Input: dimensioned drawing with shaded views. Units: mm. Origin: part minimum x, y, z. A direction names the side the tool comes from. Round coordinates to 2 decimals unless told otherwise and drop trailing zeros. Write each loop counter-clockwise with the first axis right and the second up, starting at its lowest first coordinate (ties: lowest second). Pieces come first, ordered by that corner, then holes. Notation, with made-up numbers: M 87.25,13.5 L 145.25,13.5 A23 cw 145.25,49.5 Z; hole C 65,81 d10. An arc over 180 degrees is marked long. Answer in a Markdown table with one row per item. Add a question column.
Item 1: Cut plane D-D on x = 21. Return loops of the section in (y, z).
Item 2: Contact query for flat-ended pins moving along their axis: pin 1 (1.5 mm diameter, centred on x = 55, y = 12.5, fed in from -Z); pin 2 (7 mm diameter, centred on y = 5, z = 24, fed in from -X); pin 3 (3 mm diameter, centred on x = 2, z = 3.5, fed in from -Y); pin 4 (3 mm diameter, centred on y = 1.5, z = 28, fed in from +X). Output: stop coordinate, or through.
Item 3: Mould query, pull axis X, two halves, no side actions, for the marked faces 1, 2 and 3. Classes: released by +X, released by -X, zero draft, split by the parting line, or undercut.
Item 4: Cut plane A-A on z = 30. Return loops of the section in (x, y).
Item 5: Cut plane C-C on y = 8.5. Return loops of the section in (x, z), and give its area (3 significant figures).
Item 6: Material intervals for probe 1 along Z at (x, y) = (3, 11.85); probe 2 along X at (y, z) = (11, 35); probe 3 along Z at (x, y) = (37, 5), sorted ascending.
Item 7: Set-up query: the marked faces 4 and 5. Return all of +Z, -Z, +X, -X, +Y, -Y with unobstructed straight access to the full face (end or side cutting, diameter ignored); none if empty.
Item 8: Cut plane B-B on x = 3. Return loops of the section in (y, z).
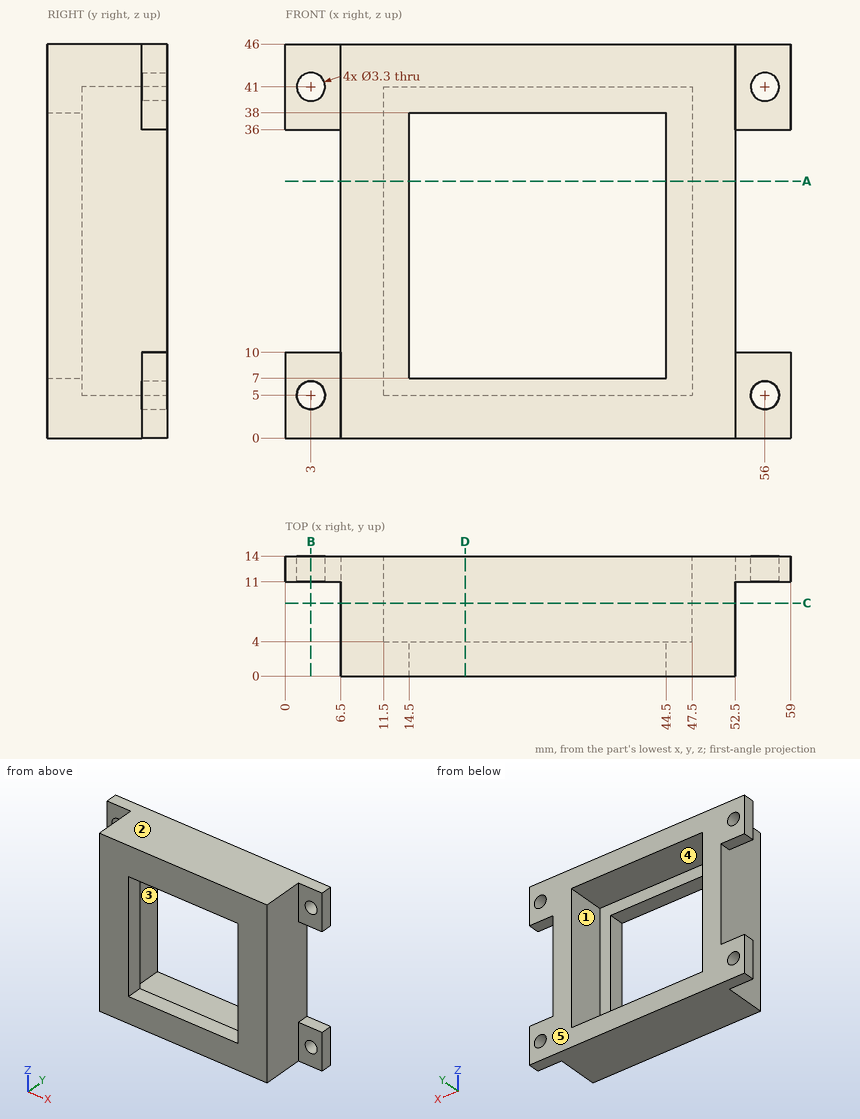
Results below:
| question | item | result |
|---|---|---|
| 1 | outline | M 0,0 L 14,0 L 14,5 L 4,5 L 4,7 L 0,7 Z; M 0,38 L 4,38 L 4,41 L 14,41 L 14,46 L 0,46 Z |
| 2 | pin 1 | z = 0 |
| 2 | pin 2 | x = 6.5 |
| 2 | pin 3 | y = 11 |
| 2 | pin 4 | x = 52.5 |
| 3 | face 1 | undercut |
| 3 | face 2 | zero draft |
| 3 | face 3 | undercut |
| 4 | outline | M 6.5,0 L 14.5,0 L 14.5,4 L 11.5,4 L 11.5,14 L 6.5,14 Z; M 44.5,0 L 52.5,0 L 52.5,14 L 47.5,14 L 47.5,4 L 44.5,4 Z |
| 5 | outline | M 6.5,0 L 52.5,0 L 52.5,46 L 6.5,46 Z; hole M 11.5,5 L 47.5,5 L 47.5,41 L 11.5,41 Z |
| 5 | area | 820 mm2 |
| 6 | probe 1 | 0 to 3.35, 6.65 to 10, 36 to 39.35, 42.65 to 46 |
| 6 | probe 2 | 6.5 to 11.5, 47.5 to 52.5 |
| 6 | probe 3 | 0 to 5, 41 to 46 |
| 7 | face 4 | +Y |
| 7 | face 5 | +Z, -Z, +X, -X, +Y |
| 8 | outline | M 11,0 L 14,0 L 14,3.35 L 11,3.35 Z; M 11,6.65 L 14,6.65 L 14,10 L 11,10 Z; M 11,36 L 14,36 L 14,39.35 L 11,39.35 Z; M 11,42.65 L 14,42.65 L 14,46 L 11,46 Z |
